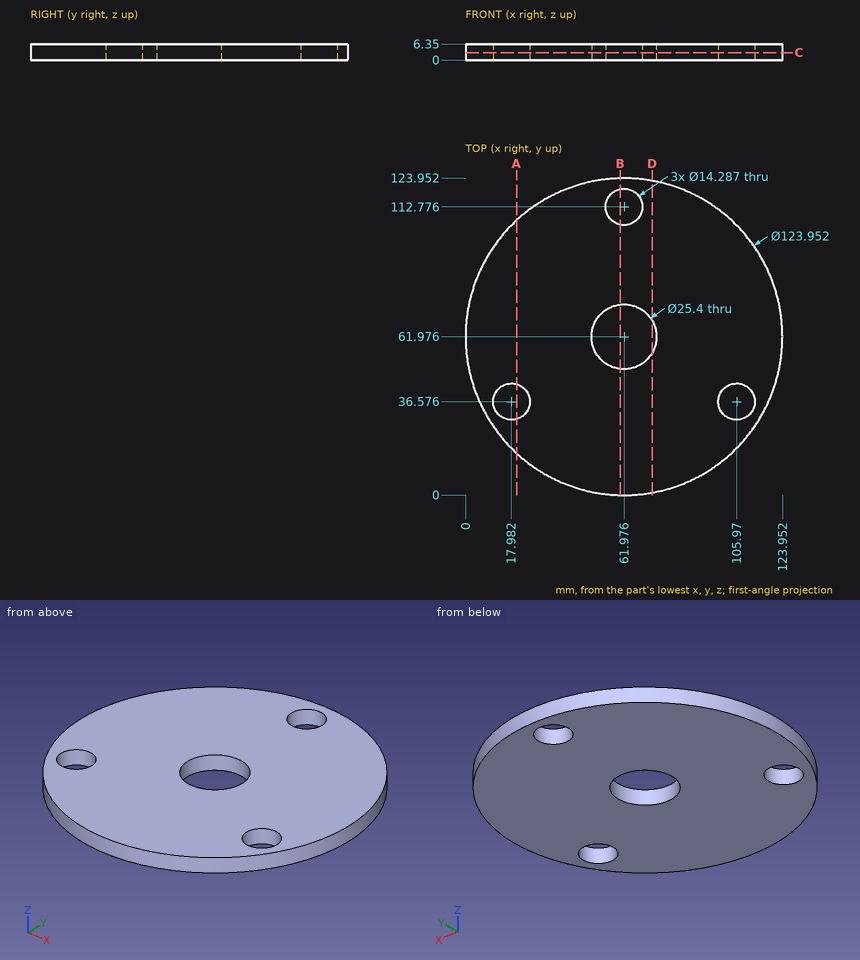
Check sheet for the drawn part. Datum: minimum x, y, z corner. Units: mm. Round coordinates to 2 decimals unless told otherwise and drop trailing zeros. Write each loop counter-clockwise with the first axis right and the second up, starting at its lowest first coordinate (ties: lowest second). Pieces come first, ordered by that corner, then holes. Notation, with made-up numbers: (19.5, 13.5) -> (50.5, 13.5) arc R19 cw to (50.5, 35.5) -> close; hole circle Ø6 at (-20, 62.25). An arc over 180 degrees is marked (long way). Put each result on its own line as item: value.
(1) Material ranges on line 1 (Y direction, x = 58, z = 5.5) (1 decimal); line 2 (Y direction, x = 57, z = 5.75); line 3 (X direction, y = 70.5, z = 3.5) (1 decimal), recorded low to high.
Values found:
line 1: y = 0.1 to 49.9, 74 to 106.8, 118.7 to 123.8
line 2: y = 0.2 to 50.29, 73.66 to 107.65, 117.9 to 123.75
line 3: x = 0.6 to 52.6, 71.4 to 123.4
(2) Sectioned sample at A-A (x = 20). Enter the section's corners in (y, z).
Values found:
outline: (16.38, 0) -> (29.72, 0) -> (29.72, 6.35) -> (16.38, 6.35) -> close; (43.43, 0) -> (107.57, 0) -> (107.57, 6.35) -> (43.43, 6.35) -> close
(3) Sectioned sample at D-D (x = 73). Enter the section's corners in (y, z).
Values found:
outline: (0.99, 0) -> (55.67, 0) -> (55.67, 6.35) -> (0.99, 6.35) -> close; (68.28, 0) -> (122.96, 0) -> (122.96, 6.35) -> (68.28, 6.35) -> close
(4) Sectioned sample at C-C (z = 3). Enter the section's corners in (x, y) (1 decimal), plus the area to 3 significant figures.
Values found:
outline: circle Ø124 at (62, 62); hole circle Ø14.3 at (18, 36.6); hole circle Ø25.4 at (62, 62); hole circle Ø14.3 at (62, 112.8); hole circle Ø14.3 at (106, 36.6)
area: 11,100 mm^2
(5) Sectioned sample at B-B (x = 60.5). Count the separate pieces of the cut face and the enclosed holes in it, plus the area to 3 significant figures.
Values found:
separate pieces: 3
enclosed holes: 0
area: 538 mm^2
(6) Go/stop test with flat-tipped pins: pin 1 Ø3 at (y, z) = (30.5, 1.5) entering from -X; pin 2 Ø1.5 at (x, y) = (77, 86) entering from -Z; pin 3 Ø2 at (y, z) = (55.5, 3.5) entering from -X; pin 4 Ø1.5 at (y, z) = (44.5, 5.5) entering from +X. Record where each tip stops, or that it passes through.
Values found:
pin 1: stops at x = 7.73
pin 2: stops at z = 0
pin 3: stops at x = 0.24
pin 4: stops at x = 121.65
